Check sheet for the modelled part. Datum: model origin and axes. Units: mm. A direction names the side the tool comes from. Round coordinates to 2 decimals unless told otherwise and drop trailing zeros. Loops run counter-clockwise (first coordinate to the right, second up) from the corner with the lowest first, then second, coordinate; pieces in that order, holes last. Notation, with made-up numbers: (0, -36.75) -> (11, -36.75) arc R23 cw to (11, -0.75) -> close; hole circle Ø6 at (52, 54). An arc over 180 degrees is marked (long way). One line per question, with ' | ' between items.
```python
from build123d import *

# Parameters (mm, degrees)
EXTRUDE_THIN1_DEPTH = 421.049210887
FILLET1_R           = 10
SKETCH_2_R          = 19.05
EXTRUDE_1_DEPTH     = 23.24974156
SKETCH_3_R          = 19.05
EXTRUDE_2_DEPTH     = 26


with BuildPart() as part:
    # Sketch1 → Extrude-Thin1 (new body, symmetric)
    with BuildSketch(Plane.XY):
        Polygon((-250.514148937, 25.753634758), (-250.514148937, 0), (440.503291061, 0), (440.503291061, 25.915671281), (446.551474959, 25.915671281), (446.551474959, -6.048183898), (-256.562332835, -6.048183898), (-256.562332835, 25.753634758), align=None)
    extrude(amount=EXTRUDE_THIN1_DEPTH, both=True)

    # Fillet1
    fillet1_edges = [part.edges().sort_by_distance(p)[0] for p in [
        (-253.538240886, 25.753634758, 421.049210887),
        (443.52738301, 25.915671281, 421.049210887),
        (-253.538240886, 25.753634758, -421.049210887),
        (443.52738301, 25.915671281, -421.049210887),
    ]]
    fillet(fillet1_edges, radius=FILLET1_R)

    # 草图2 → 凸台-拉伸1 (add)
    with BuildSketch(Plane(origin=(0, -6.048183898, 0), x_dir=(-1, 0, 0), z_dir=(0, -1, 0))):
        with Locations((-360.164689426, 358.012657815)):
            Circle(SKETCH_2_R)
    extrude(amount=EXTRUDE_1_DEPTH)

    # 草图3 → 凸台-拉伸2 (add)
    with BuildSketch(Plane(origin=(0, -6.048183898, 0), x_dir=(-1, 0, 0), z_dir=(0, -1, 0))):
        with Locations((175.410326922, -359.721177401)):
            Circle(SKETCH_3_R)
    extrude(amount=EXTRUDE_2_DEPTH)


solid = part.part
```
(1) Sectioned sample at C-C, the plane x = 127.5. Record the cut outline in (y, z).
Answer:
outline: (-6.05, -421.05) -> (0, -421.05) -> (0, 421.05) -> (-6.05, 421.05) -> close
(2) Sectioned sample at B-B, the plane x = -181. Record the cut outline in (y, z).
Answer:
outline: (-32.05, 341.51) -> (-6.05, 341.51) -> (-6.05, -421.05) -> (0, -421.05) -> (0, 421.05) -> (-6.05, 421.05) -> (-6.05, 377.93) -> (-32.05, 377.93) -> close
(3) Go/stop test with flat-tipped pins: pin 1 (10 mm diameter, centred on x = 111.5, z = 148.5, fed in from -Y); pin 2 (5 mm diameter, centred on x = -254, z = -198.5, fed in from +Y). Record where each tip stops, or that it passes through.
Answer:
pin 1: stops at y = -6.05 | pin 2: stops at y = 25.75
(4) Sectioned sample at A-A, the plane z = 109. Record the cut outline in (x, y).
Answer:
outline: (-256.56, -6.05) -> (446.55, -6.05) -> (446.55, 25.92) -> (440.5, 25.92) -> (440.5, 0) -> (-250.51, 0) -> (-250.51, 25.75) -> (-256.56, 25.75) -> close
(5) Set-up check for faces 1 (the face through (-171.28, -18.87, 378.32)), 2 (the face through (90, 0, 6)), 3 (the face through (97, -2, 421.049)): record each of +Z, -Z, +X, -X, +Y, -Y from which the full face is reachable in a straight line by a thin tool's end or side.
Answer:
face 1: -Y | face 2: +Z, -Z, +Y | face 3: +Z, +X, -X, +Y, -Y
(6) Scan lines: probe 1 along X at (y, z) = (23, 122); probe 2 along Y at (x, z) = (398, 338); probe 3 along Z at (x, y) = (372, -12.5). Record each from-to range of solid material in increasing order.
Answer:
probe 1: x = -256.56 to -250.51, 440.5 to 446.55 | probe 2: y = -6.05 to 0 | probe 3: z = -372.94 to -343.09
(7) Mould release check, pull along X, two halves, no side actions. Record for faces 4 (the face through (440.503, 13, 6)), 5 (the face through (446.551, 10, 6)), 6 (the face through (349.924, -17.51, -374.076)): +X half, -X half, draft (parallel to the pull), parting line (faces both ways), or undercut.
Answer:
face 4: undercut | face 5: +X half | face 6: parting line
